Input: part model. Units: mm. Frame: model coordinates. A direction names the side the tool comes from. Coordinates: 2 decimals unless noted, no trailing zeros. Order: outer loops, then holes, each group sorted by start corner. A loop starts at its lowest first (then second) coordinate and runs counter-clockwise, first axis right, second up. Notation, with made-up numbers: M 77,75.5 L 114,75.5 A12 ccw 114,79.5 Z; hole C 43.25,79 d8. An arc over 180 degrees is marked long. One line per item, written item: value.
```python
from build123d import *

# Parameters (mm, degrees)
BOSS_EXTRU_1_DEPTH      = 10
ESQUISSE2_R             = 4.5
BOSS_EXTRU_2_DEPTH      = 5
ESQUISSE3_R             = 1.525
ESQUISSE3_R_2           = 5
ENL_V_MAT_EXTRU_1_DEPTH = 221.29310456


with BuildPart() as part:
    # Esquisse1 → Boss.-Extru.1 (new body)
    with BuildSketch(Plane.XY):
        with BuildLine():
            Line((-55, 32.372583002), (-22.627416998, 0))
            Line((-22.627416998, 0), (0, 0))
            Line((0, 0), (0, 22.627416998))
            Line((0, 22.627416998), (-32.372583002, 55))
            Line((-32.372583002, 55), (-115.811183182, 138.43860018))
            ThreePointArc((-115.811183182, 138.43860018), (-115.660488879, 137.027953457), (-115.610173055, 135.610173055))
            ThreePointArc((-115.610173055, 135.610173055), (-122.506138228, 120.501093955), (-138.43860018, 115.811183182))
            Line((-138.43860018, 115.811183182), (-55, 32.372583002))
        make_face()
        with BuildLine():
            ThreePointArc((-115.811183182, 138.43860018), (-149.752308679, 149.752308679), (-138.43860018, 115.811183182))
            Line((-138.43860018, 115.811183182), (-146.923881554, 124.296464556))
            Line((-146.923881554, 124.296464556), (-124.296464556, 146.923881554))
            Line((-124.296464556, 146.923881554), (-115.811183182, 138.43860018))
        make_face()
        with BuildLine():
            Line((-146.923881554, 124.296464556), (-138.43860018, 115.811183182))
            ThreePointArc((-138.43860018, 115.811183182), (-122.506138228, 120.501093955), (-115.610173055, 135.610173055))
            ThreePointArc((-115.610173055, 135.610173055), (-115.660488879, 137.027953457), (-115.811183182, 138.43860018))
            Line((-115.811183182, 138.43860018), (-124.296464556, 146.923881554))
            Line((-124.296464556, 146.923881554), (-146.923881554, 124.296464556))
        make_face()
    extrude(amount=BOSS_EXTRU_1_DEPTH)

    # Esquisse2 → Boss.-Extru.2 (add)
    with BuildSketch(Plane(origin=(0, 0, 0), x_dir=(-1, 0, 0), z_dir=(0, 0, -1))):
        with Locations(Location((31.819805153, 31.819805153, 0), (0, 0, 180))):
            Circle(ESQUISSE2_R)
        with Locations(Location((14.142135624, 14.142135624, 0), (0, 0, 180))):
            Circle(ESQUISSE2_R)
    extrude(amount=BOSS_EXTRU_2_DEPTH)

    # Esquisse3 → Enlèv. mat.-Extru.1 (cut, through all)
    with BuildSketch(Plane(origin=(0, 0, 0), x_dir=(-1, 0, 0), z_dir=(0, 0, -1))):
        with Locations((135.610173055, 145.110173055)):
            Circle(ESQUISSE3_R)
        with Locations((145.110173055, 135.610173055)):
            Circle(ESQUISSE3_R)
        with Locations((135.610173055, 126.110173055)):
            Circle(ESQUISSE3_R)
        with Locations((126.110173055, 135.610173055)):
            Circle(ESQUISSE3_R)
        with Locations((84.852813742, 84.852813742)):
            Circle(ESQUISSE3_R_2)
    extrude(amount=-ENL_V_MAT_EXTRU_1_DEPTH, mode=Mode.SUBTRACT)


solid = part.part
```
(1) First-contact query: pin 1 (2.5 mm diameter, centred on x = -145.11, y = 135.61, fed in from -Z); pin 2 (6 mm diameter, centred on x = -139.5, z = 3, fed in from -Y); pin 3 (3 mm diameter, centred on y = 116.5, z = 4.5, fed in from +X); pin 4 (6 mm diameter, centred on x = -122, y = 97, fed in from -Z). Flat tips, straight axial feed; report the tip coordinate or a pass-through.
Data:
pin 1: passes through
pin 2: stops at y = 113.87
pin 3: stops at x = -92.37
pin 4: stops at z = 0
(2) Cut plane C-C on x = -32. Output: boundary loops of the cut face in (y, z), plus the area to 3 significant figures.
Data:
outline: M 9.37,0 L 27.32,0 L 27.32,-5 L 36.32,-5 L 36.32,0 L 54.63,0 L 54.63,10 L 9.37,10 Z
area: 498 mm2
(3) Access query for faces 5 (the flat face through (-32, 32, -5)), 6 (the cylindrical face through (-36.315, 31.622, -2.465)). Directions: +Z, -Z, +X, -X, +Y, -Y. A direction counts if a zero-diameter tool reaches every point of the face in a straight line with its end or side. Return the directions, or none.
Data:
face 5: -Z, +X, -X, +Y, -Y
face 6: -Z
(4) Ray query, line 1 (X direction, y = 31.5, z = -1.5); line 2 (Z direction, x = -74, y = 85.5); line 3 (Y direction, x = -82, z = 0.5). Return the intervals inside material, ascending. Write a range as from..to.
Data:
line 1: x = -36.31..-27.33
line 2: z = 0..10
line 3: y = 59.37..80.75, 88.96..104.63
(5) Draft query along Y for faces 1 (the cylindrical face through (-149.31, 150.18, 4.93)), 2 (the cylindrical face through (-83.77, 79.97, 4.93)), 3 (the flat face through (-57.09, 79.72, 4.93)), 4 (the flat face through (-81.344, 58.716, 4.93)). Return one class per face: released by +Y, released by -Y, zero draft, split by the parting line, or undercut.
Data:
face 1: split by the parting line
face 2: undercut
face 3: released by +Y
face 4: released by -Y
(6) Cut plane B-B on z = 3. Output: boundary loops of the cut face in (x, y) (3 decimals).
Data:
outline: M -138.439,115.811 L -22.627,0 L 0,0 L 0,22.627 L -115.811,138.439 A20 ccw long Z; hole C -145.11,135.61 d3.05; hole C -135.61,126.11 d3.05; hole C -135.61,145.11 d3.05; hole C -126.11,135.61 d3.05; hole C -84.853,84.853 d10
(7) Cut plane A-A on x = -84. Output: boundary loops of the cut face in (y, z), plus the area to 3 significant figures.
Data:
outline: M 61.37,0 L 79.93,0 L 79.93,10 L 61.37,10 Z; M 89.78,0 L 106.63,0 L 106.63,10 L 89.78,10 Z
area: 354 mm2
(8) Cut plane D-D on y = 73. Output: boundary loops of the cut face in (x, z), plus the area to 3 significant figures.
Data:
outline: M -95.63,0 L -50.37,0 L -50.37,10 L -95.63,10 Z
area: 453 mm2
